from build123d import *

# Parameters (mm, degrees)
SKETCH_1_R          = 2.5
SKETCH_1_W          = 1
SKETCH_1_H          = 1.7
EXTRUDE_1_DEPTH     = 1.1
SKETCH_2_W          = 1
SKETCH_2_H          = 1.7
CUT_EXTRUDE_1_DEPTH = 1.8
SKETCH_3_R          = 0.5
EXTRUDE_2_DEPTH     = 1.2
CHAMFER_1_SIZE      = 0.1


with BuildPart() as part:
    # 草图1 → 凸台-拉伸1 (new, symmetric)
    # profile 1 of 5: a face of its own
    with BuildSketch(Plane(origin=(0, 0, 0), x_dir=(1, 0, 0), z_dir=(0, 1, 0))):
        with BuildLine():
            Line((0, 1.5), (0, 6.5))
            ThreePointArc((0, 6.5), (5.5, 12), (11, 6.5))
            Line((11, 6.5), (11, 1.5))
            ThreePointArc((11, 1.5), (10.560660172, 0.439339828), (9.5, 0))
            Line((9.5, 0), (1.5, 0))
            ThreePointArc((1.5, 0), (0.439339828, 0.439339828), (0, 1.5))
        make_face()
        with Locations(Location((5.5, 6.5, 0), (0, 0, 270))):
            Circle(SKETCH_1_R, mode=Mode.SUBTRACT)
    # profile 2 of 5: a face of its own
    with BuildSketch(Plane(origin=(0, 0, 0), x_dir=(1, 0, 0), z_dir=(0, 1, 0))):
        with Locations((3, -0.85)):
            Rectangle(SKETCH_1_W, SKETCH_1_H)
    # profile 3 of 5: a face of its own
    with BuildSketch(Plane(origin=(0, 0, 0), x_dir=(1, 0, 0), z_dir=(0, 1, 0))):
        with Locations((5.5, -0.85)):
            Rectangle(SKETCH_1_W, SKETCH_1_H)
    # profile 4 of 5: a face of its own
    with BuildSketch(Plane(origin=(0, 0, 0), x_dir=(1, 0, 0), z_dir=(0, 1, 0))):
        with Locations((8, -0.85)):
            Rectangle(SKETCH_1_W, SKETCH_1_H)
    # profile 5 of 5: a face of its own
    with BuildSketch(Plane(origin=(0, 0, 0), x_dir=(1, 0, 0), z_dir=(0, 1, 0))):
        with Locations((5.5, 12.827225575)):
            Rectangle(SKETCH_1_W, SKETCH_1_H)
    extrude(amount=EXTRUDE_1_DEPTH, both=True)

    # 草图2 → 切除-拉伸1 (cut)
    with BuildSketch(Plane(origin=(0, 1.1, 0), x_dir=(1, 0, 0), z_dir=(0, 1, 0))):
        with Locations((5.5, 12.827225575)):
            Rectangle(SKETCH_2_W, SKETCH_2_H)
        with Locations((3, -0.85)):
            Rectangle(SKETCH_2_W, SKETCH_2_H)
        with Locations((5.5, -0.85)):
            Rectangle(SKETCH_2_W, SKETCH_2_H)
        with Locations((8, -0.85)):
            Rectangle(SKETCH_2_W, SKETCH_2_H)
    extrude(amount=-CUT_EXTRUDE_1_DEPTH, mode=Mode.SUBTRACT)

    # 草图3 → 凸台-拉伸2 (add)
    with BuildSketch(Plane.XZ.offset(1.1)):
        with Locations(Location((1.25, -1, 0), (0, 0, 90))):
            Circle(SKETCH_3_R)
        with Locations(Location((9.75, -1, 0), (0, 0, 90))):
            Circle(SKETCH_3_R)
    extrude(amount=EXTRUDE_2_DEPTH)

    # 倒角1
    chamfer_1_edges = [part.edges().sort_by_distance(p)[0] for p in [
        (1.25, -2.3, -1.5),
        (9.75, -2.3, -1.5),
    ]]
    chamfer(chamfer_1_edges, length=CHAMFER_1_SIZE)


solid = part.part
For this review, take the finished solid that the model builds, in its own axes (mm). A direction names the side the tool comes from. Round coordinates to 2 decimals unless told otherwise and drop trailing zeros. Order: outer loops, then holes, each group sorted by start corner. A loop starts at its lowest first (then second) coordinate and runs counter-clockwise, first axis right, second up. Notation, with made-up numbers: (-32.75, 33.5) -> (-3.75, 33.5) arc R11 ccw to (-3.75, 40.5) -> close; hole circle Ø1 at (25, -4). An arc over 180 degrees is marked (long way). Write item = value, one per line. Start each with the question number.
1) Tool access review of faces 5 (the face through (5, 1.1, -3)), 6 (the face through (3, -0.7, 1)), 7 (the face through (5.5, -0.7, -12.8)): name each direction out of +Z, -Z, +X, -X, +Y, -Y from which nothing blocks a thin tool from reaching the whole face with its end or side.
2) Take a section at A-A on z = -5. State the section outline as (x, y) points, plus the area to 3 significant figures.
3) Take a section at D-D on y = -1.65. State the section outline as (x, z) points.
4) Insertion check: pin 1 (1.5 mm diameter, centred on y = 0, z = -8, fed in from -X); pin 2 (1.1 mm diameter, centred on x = 3.5, y = 0.5, fed in from +Z); pin 3 (0.8 mm diameter, centred on x = 8, z = 1, fed in from +Y). Each pin has a flat end and moves straight along its axis. Give the tip position at first contact, or say it passes through.
5) To check wall thickness, follow line 1 (X direction, y = 0.6, z = -6.5); line 2 (Y direction, x = 1.5, z = -4); line 3 (X direction, y = 0.5, z = -8.25). State the ranges of each line that lie inside material, in increasing order. Write a range as from..to.
6) Take a section at B-B on y = 0.1. State the section outline as (x, z) points, plus the area to 3 significant figures.
7) Take a section at C-C on x = 5.5. State the section outline as (y, z) points.
8) The part is to be moulded in two halves that separate along X. For faces 1 (the face through (1.55, -1.64, -1.4)), 2 (the face through (10.238, -1.642, -1.108)), 3 (the face through (5.5, -0.7, 0.8)), 4 (the face through (1.4, 0.015, -10.166)), say which applies: +X half, -X half, draft (parallel to the pull), parting line (faces both ways), or undercut.
Verdict:
q1.face_5 = +Z, -Z, +X, -X, +Y
q1.face_6 = +Z, +X, -X, +Y
q1.face_7 = -Z, +X, -X, +Y
q2.outline = (0, -1.1) -> (3.5, -1.1) -> (3.5, 1.1) -> (0, 1.1) -> close; (7.5, -1.1) -> (11, -1.1) -> (11, 1.1) -> (7.5, 1.1) -> close
q2.area = 15.4 mm2
q3.outline = circle Ø1 at (1.25, -1); circle Ø1 at (9.75, -1)
q4.pin_1 = 0.05
q4.pin_2 = 0
q4.pin_3 = -0.7
q5.line_1 = 0..3, 8..11
q5.line_2 = -1.1..1.1
q5.line_3 = 0.29..3.71, 7.29..10.71
q6.outline = (0, -6.5) arc R5.5 ccw to (5, -11.98) -> (6, -11.98) arc R5.5 ccw to (11, -6.5) -> (11, -1.5) arc R1.5 ccw to (9.5, 0) -> (1.5, 0) arc R1.5 ccw to (0, -1.5) -> close; hole circle Ø5 at (5.5, -6.5)
q6.area = 98.4 mm2
q7.outline = (-1.1, -13.68) -> (-0.7, -13.68) -> (-0.7, -11.98) -> (1.1, -11.98) -> (1.1, -9) -> (-1.1, -9) -> close; (-1.1, -4) -> (1.1, -4) -> (1.1, 0) -> (-0.7, 0) -> (-0.7, 1.7) -> (-1.1, 1.7) -> close
q8.face_1 = undercut
q8.face_2 = undercut
q8.face_3 = draft
q8.face_4 = -X half
